from build123d import *

# Parameters (mm, degrees)
CUT_EXTRUDE1_DEPTH = 136.422799192
SHELL1_T           = -0.396875
SKETCH3_R          = 3.175
CUT_EXTRUDE2_DEPTH = 136.114809977


with BuildPart() as part:
    # Sketch1 → Revolve1 (revolve)
    with BuildSketch(Plane.XY, mode=Mode.PRIVATE) as revolve1_sk:
        Polygon((0, 105.171875), (60.325, 105.171875), (60.325, 0), (59.928125, 0), (0, 0), align=None)
    revolve(revolve1_sk.sketch.rotate(Axis((0, 0, 0), (0, 1, 0)), 90), axis=Axis((0, 0, 0), (0, 1, 0)))

    # Sketch2 → Cut-Extrude1 (cut, through all)
    with BuildSketch(Plane(origin=(0, 105.171875, 0), x_dir=(1, 0, 0), z_dir=(0, 1, 0))):
        with BuildLine():
            ThreePointArc((43.664470656, 23.849143646), (9.525, 0), (43.664470656, -23.849143646))
            ThreePointArc((43.664470656, -23.849143646), (50.360604205, -25.718912301), (50.717833444, -32.662011508))
            ThreePointArc((50.717833444, -32.662011508), (60.325, 0), (50.717833444, 32.662011508))
            ThreePointArc((50.717833444, 32.662011508), (50.360604205, 25.718912301), (43.664470656, 23.849143646))
        make_face()
    extrude(amount=-CUT_EXTRUDE1_DEPTH, mode=Mode.SUBTRACT)

    # Shell1
    shell1_openings = [part.faces().sort_by_distance(p)[0] for p in [
        (-8.714175157, 0, 0),
    ]]
    offset(amount=SHELL1_T, openings=shell1_openings, kind=Kind.INTERSECTION)

    # Sketch3 → Cut-Extrude2 (cut, through all)
    with BuildSketch(Plane.XZ.offset(-104.775)):
        with Locations(Location((0, 0, 0), (0, 0, 270))):
            Circle(SKETCH3_R)
    extrude(amount=-CUT_EXTRUDE2_DEPTH, mode=Mode.SUBTRACT)


solid = part.part
Verification items for the finished model (mm, model axes). A direction names the side the tool comes from. Coordinates: 2 decimals unless noted, no trailing zeros. Loops run counter-clockwise (first coordinate to the right, second up) from the corner with the lowest first, then second, coordinate; pieces in that order, holes last. Notation, with made-up numbers: (35, 4) -> (41, 4) arc R13 cw to (41, 21) -> close; hole circle Ø11 at (-10.75, 30.25). An arc over 180 degrees is marked (long way). Answer as a JSON object with one key per item and string values. Group by question number.
Item 1: Sectioned sample at D-D on x = -30. Record the boundary of the cut face in (y, z) (3 decimals).
Item 2: Tool access check on faces 1 (the cylindrical face through (50.11, 53.12, -26.04)), 2 (the cylindrical face through (9.534, 53.322, -0.683)). Record the directions out of +Z, -Z, +X, -X, +Y, -Y that give a thin tool (end or side, any length) a straight path to the whole face; none if there is none.
Item 3: Scan lines: probe 1 along X at (y, z) = (25, 0) (3 decimals); probe 2 along Z at (x, y) = (11.5, 79) (3 decimals); probe 3 along Z at (x, y) = (0, 69) (3 decimals). Record each from-to range of solid material in increasing order.
Item 4: Depth check by flat-ended pin: pin 1 (1.5 mm diameter, centred on y = 44, z = -38.5, fed in from +X); pin 2 (5 mm diameter, centred on x = -15, y = 81, fed in from +Z); pin 3 (10 mm diameter, centred on x = 23.5, y = 23, fed in from -Z); pin 4 (12 mm diameter, centred on x = 20, z = -10.5, fed in from -Y). Enter the tip coordinate at first touch or a pass-through.
Item 5: Sectioned sample at A-A on x = 0. Record the boundary of the cut face in (y, z) (3 decimals).
Item 6: Mould release check, pull along Z, two halves, no side actions. Record for faces 3 (the cylindrical face through (-60.286, 51.85, -2.17)), 4 (the cylindrical face through (9.137, 53.121, -0.694)), 5 (the flat face through (-5, 105.172, -1)): +Z half, -Z half, draft (parallel to the pull), parting line (faces both ways), or undercut.
Item 7: Sectioned sample at B-B on z = 0. Record the boundary of the cut face in (x, y) (3 decimals).
Evaluation:
{
 "1": {"outline": "(0, -52.336) -> (105.172, -52.336) -> (105.172, 52.336) -> (0, 52.336) -> (0, 51.879) -> (104.775, 51.879) -> (104.775, -51.879) -> (0, -51.879) -> close"},
 "2": {"face 1": "-Y", "face 2": "+Y, -Y"},
 "3": {"probe 1": "x = -60.325 to -59.928, 9.128 to 9.525", "probe 2": "z = -59.219 to -58.814, -10.805 to -9.82, 9.82 to 10.805, 58.814 to 59.219", "probe 3": "z = -60.325 to -59.928, 59.928 to 60.325"},
 "4": {"pin 1": "stops at x = 47.05", "pin 2": "stops at z = 59.02", "pin 3": "stops at z = -57.42", "pin 4": "passes through"},
 "5": {"outline": "(0, -60.325) -> (105.172, -60.325) -> (105.172, -3.175) -> (104.775, -3.175) -> (104.775, -59.928) -> (0, -59.928) -> close; (0, 59.928) -> (104.775, 59.928) -> (104.775, 3.175) -> (105.172, 3.175) -> (105.172, 60.325) -> (0, 60.325) -> close"},
 "6": {"face 3": "parting line", "face 4": "undercut", "face 5": "draft"},
 "7": {"outline": "(-60.325, 0) -> (-59.928, 0) -> (-59.928, 104.775) -> (-3.175, 104.775) -> (-3.175, 105.172) -> (-60.325, 105.172) -> close; (3.175, 104.775) -> (9.128, 104.775) -> (9.128, 0) -> (9.525, 0) -> (9.525, 105.172) -> (3.175, 105.172) -> close"}
}
